Geometry check sheet. Reference: the model listing, model coordinates, mm. A direction names the side the tool comes from. Round coordinates to 2 decimals unless told otherwise and drop trailing zeros. Order: outer loops, then holes, each group sorted by start corner. A loop starts at its lowest first (then second) coordinate and runs counter-clockwise, first axis right, second up. Notation, with made-up numbers: (80, -12) -> (108, -12) arc R26 cw to (108, 22) -> close; hole circle Ø8 at (63, 28.25). An arc over 180 degrees is marked (long way). Use a Markdown table: item, result. Add a question column.
Item 1: Gauge pin test, flat ends, axial feed: pin 1 Ø3 at (x, y) = (-85, -45) entering from +Z; pin 2 Ø25 at (x, y) = (20, 1) entering from -Z; pin 3 Ø2.5 at (x, y) = (-76.5, 5.5) entering from -Z. Record the tip position at first contact, or that the pin passes through.
Item 2: Sectioned sample at B-B, the plane z = -237.5. Record the cut outline in (x, y), and give its area (3 significant figures).
Item 3: Set-up check for faces 5 (the flat face through (75, 0, -260)), 6 (the cylindrical face through (4.38, 8.43, -69.79)), 7 (the flat face through (125, 73, -516)): record each of +Z, -Z, +X, -X, +Y, -Y from which the full face is reachable in a straight line by a thin tool's end or side.
Item 4: Sectioned sample at A-A, the plane x = 0. State how many separate pieces and enclosed holes the cut face has, and give its area (3 significant figures).
Item 5: Sectioned sample at D-D, the plane y = 33.5. Record the cut outline in (x, z).
Item 6: Material ranges on probe 1 along X at (y, z) = (6, -260); probe 2 along Y at (x, z) = (39.5, -504); probe 3 along Z at (x, y) = (26.5, -2.5), recorded low to high. Write a range as [from, to].
Item 7: Mould release check, pull along Z, two halves, no side actions. Record for faces 1 (the cylindrical face through (11.923, -3.755, -52.465)), 2 (the flat face through (-75, 0, -260)), 3 (the flat face through (-125, 0, -243)), 4 (the flat face through (2, 85, -540)): pulls with the +Z half, pulls with the -Z half, needs draft (parallel to the pull), parting line crosses it, or undercut.
from build123d import *

# Parameters (mm, degrees)
F0_W      = 150
F0_H      = 415
F1_DEPTH  = 25
F3_DEPTH  = 125
F5_DEPTH  = 125
F6_R      = 9.5
F7_DEPTH  = 35
F8_R      = 12.5
F9_DEPTH  = 5
F10_R     = 9.5
F11_DEPTH = 30
F12_R     = 3.5
F13_DEPTH = 30


with BuildPart() as f1:
    # F0 (on Front) → F1 (new body, symmetric)
    with BuildSketch(Plane.XZ):
        Polygon((125, -540), (125, 0), (-125, 0), (-125, -540), (-75, -540), (-75, -515), (75, -515), (75, -540), align=None)
        with Locations((0, -257.5)):
            Rectangle(F0_W, F0_H, mode=Mode.SUBTRACT)
    extrude(amount=F1_DEPTH, both=True)

    # F2 (on Front) → F3 (join, symmetric)
    with BuildSketch(Plane.XZ):
        Polygon((-125, -493), (-128, -493), (-128, -543), (-78, -543), (-78, -540), (-125, -540), align=None)
        Polygon((78, -540), (78, -543), (128, -543), (128, -493), (125, -493), (125, -540), align=None)
    extrude(amount=F3_DEPTH, both=True)

    # F4 (on Right) → F5 (join, symmetric)
    with BuildSketch(Plane.YZ):
        Polygon((125, -543), (125, -493), (122, -493), (122, -540), (75, -540), (75, -543), align=None)
        Polygon((-122, -540), (-122, -493), (-125, -493), (-125, -543), (-75, -543), (-75, -540), align=None)
    extrude(amount=F5_DEPTH, both=True)

    # F6 (on face) → F7 (join)
    with BuildSketch(Plane(origin=(0, 0, -50), x_dir=(1, 0, 0), z_dir=(0, 0, -1))):
        Circle(F6_R)
    extrude(amount=F7_DEPTH)

    # F8 (on face) → F9 (join)
    with BuildSketch(Plane(origin=(0, 0, -50), x_dir=(1, 0, 0), z_dir=(0, 0, -1))):
        Circle(F8_R)
    extrude(amount=F9_DEPTH)

    # F10 (on face) → F11 (join)
    with BuildSketch(Plane.XY.offset(-465)):
        Circle(F10_R)
    extrude(amount=F11_DEPTH)

    # F12 (on Front) → F13 (cut, symmetric)
    with BuildSketch(Plane.XZ):
        with Locations((-100, -260)):
            Circle(F12_R)
        with Locations((100, -260)):
            Circle(F12_R)
    extrude(amount=F13_DEPTH, both=True, mode=Mode.SUBTRACT)


solid = f1.part
Found:
| question | item | result |
|---|---|---|
| 1 | pin 1 | stops at z = -540 |
| 1 | pin 2 | stops at z = -515 |
| 1 | pin 3 | stops at z = -540 |
| 2 | outline | (-125, -25) -> (-75, -25) -> (-75, 25) -> (-125, 25) -> close; (75, -25) -> (125, -25) -> (125, 25) -> (75, 25) -> close |
| 2 | area | 5,000 mm2 |
| 3 | face 5 | +Y, -Y |
| 3 | face 6 | none |
| 3 | face 7 | +Z |
| 4 | separate pieces | 4 |
| 4 | enclosed holes | 0 |
| 4 | area | 6,850 mm2 |
| 5 | outline | (-128, -543) -> (-78, -543) -> (-78, -540) -> (-125, -540) -> (-125, -493) -> (-128, -493) -> close; (78, -543) -> (128, -543) -> (128, -493) -> (125, -493) -> (125, -540) -> (78, -540) -> close |
| 6 | probe 1 | x = [-125, -103.5], [-96.5, -75], [75, 96.5], [103.5, 125] |
| 6 | probe 2 | y = [-125, -122], [-25, 25], [122, 125] |
| 6 | probe 3 | z = [-515, -465], [-50, 0] |
| 7 | face 1 | undercut |
| 7 | face 2 | undercut |
| 7 | face 3 | needs draft |
| 7 | face 4 | pulls with the +Z half |
